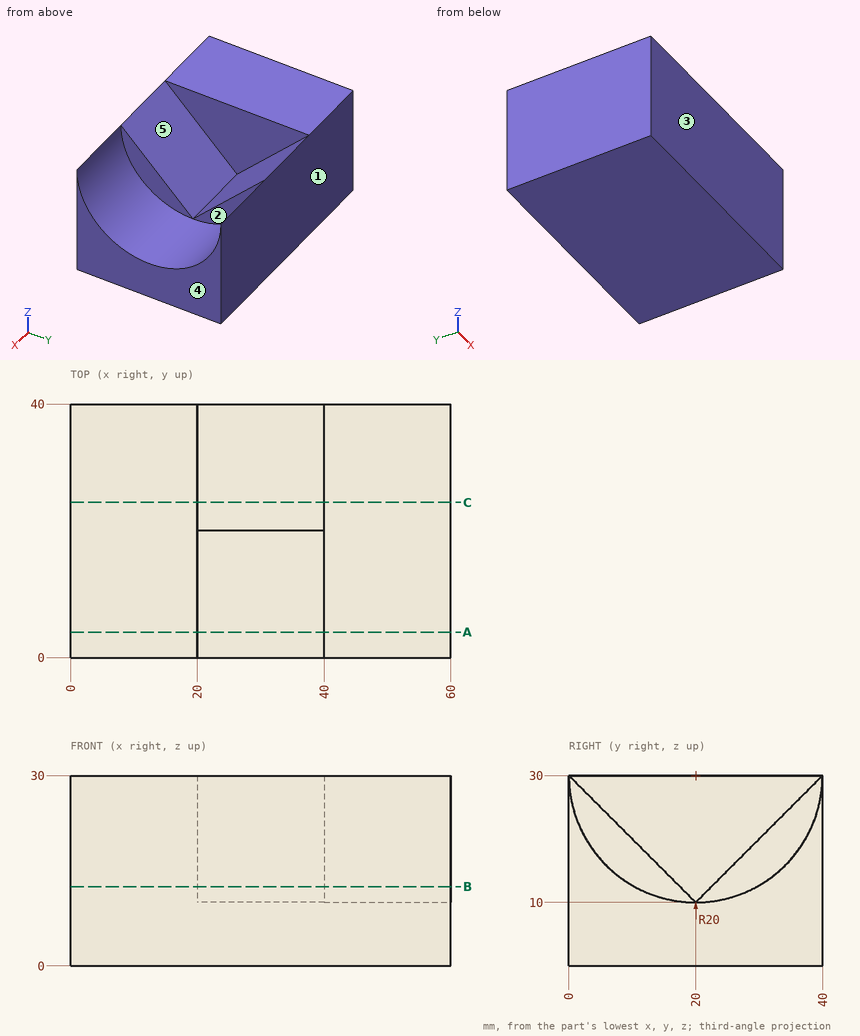
Geometry check sheet. Reference: drawing and pictorial views, mm from the part's lowest x, y, z. A direction names the side the tool comes from. Round coordinates to 2 decimals unless told otherwise and drop trailing zeros. Loops run counter-clockwise (first coordinate to the right, second up) from the corner with the lowest first, then second, coordinate; pieces in that order, holes last.
1. Sectioned sample at B-B on z = 12.5. Record the boundary of the cut face in (x, y), and give its area (3 significant figures).
2. Mould release check, pull along Y, two halves, no side actions. Record for the marked faces 3, 4 and 5: released by +Y, released by -Y, zero draft, split by the parting line, or undercut.
3. Sectioned sample at A-A on y = 4. Record the boundary of the cut face in (x, z).
4. Gauge pin test, flat ends, axial feed: pin 1 Ø12 at (x, y) = (37.5, 16) entering from +Z; pin 2 Ø6 at (y, z) = (33, 26) entering from +X; pin 3 Ø3 at (y, z) = (30.5, 26) entering from +X. Record the tip position at first contact, or that the pin passes through.
5. Set-up check for the marked faces 1 and 2: record each of +Z, -Z, +X, -X, +Y, -Y from which the full face is reachable in a straight line by a thin tool's end or side.
6. Sectioned sample at C-C on y = 24.5. Record the boundary of the cut face in (x, z), and give its area (3 significant figures).
7. Scan lines: probe 1 along X at (y, z) = (34.5, 24); probe 2 along Y at (x, z) = (53, 13); probe 3 along Y at (x, z) = (41, 14.5). Record each from-to range of solid material in increasing order.
Recorded:
1. outline: (0, 0) - (60, 0) - (60, 10.32) - (40, 10.32) - (40, 17.5) - (20, 17.5) - (20, 22.5) - (40, 22.5) - (40, 29.68) - (60, 29.68) - (60, 40) - (0, 40) - close
1. area: 1,910 mm2
2. face 3: released by -Y
2. face 4: zero draft
2. face 5: undercut
3. outline: (0, 0) - (60, 0) - (60, 18) - (40, 18) - (40, 26) - (20, 26) - (20, 30) - (0, 30) - close
4. pin 1: stops at z = 20
4. pin 2: stops at x = 40
4. pin 3: stops at x = 20
5. face 1: +Z, -Z, +X, -X, +Y
5. face 2: +Z, +X
6. outline: (0, 0) - (60, 0) - (60, 10.51) - (40, 10.51) - (40, 14.5) - (20, 14.5) - (20, 30) - (0, 30) - close
6. area: 1,100 mm2
7. probe 1: x = 0 to 40
7. probe 2: y = 0 to 9.46, 30.54 to 40
7. probe 3: y = 0 to 7.36, 32.64 to 40
